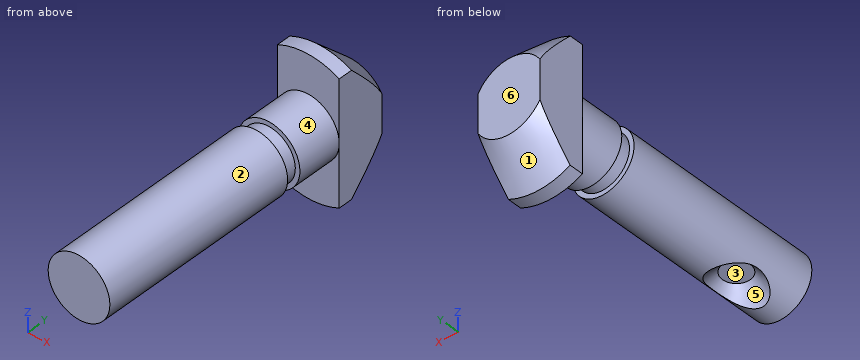
from build123d import *

# Parameters (mm, degrees)
SKETCH_3_W          = 7.345326746
SKETCH_3_H          = 8.819653772
SKETCH_3_W_2        = 8.702196558
SKETCH_3_H_2        = 9.976983905
CUT_EXTRUDE_1_DEPTH = 50


with BuildPart() as part:
    # 草图1 → 旋转1 (revolve)
    with BuildSketch(Plane.XY, mode=Mode.PRIVATE) as revolve_1_sk:
        Polygon((3.95, 33.2), (0, 33.2), (0, 0), (3.35, 0), (3.35, 21.7), (2.85, 21.7), (2.85, 23.2), (3.35, 23.2), (3.35, 28), (7.5, 28), (7.5, 29.5), align=None)
    revolve(revolve_1_sk.sketch.rotate(Axis((0, 33.2, 0), (0, 1, 0)), 270), axis=Axis((0, 33.2, 0), (0, 1, 0)))

    # 草图3 → 切除-拉伸1 (cut, symmetric)
    with BuildSketch(Plane.XY):
        with Locations((-7.022663373, 29.230861624)):
            Rectangle(SKETCH_3_W, SKETCH_3_H)
        with Locations((7.701098279, 29.530171142)):
            Rectangle(SKETCH_3_W_2, SKETCH_3_H_2)
    extrude(amount=CUT_EXTRUDE_1_DEPTH, both=True, mode=Mode.SUBTRACT)

    # 草图4 → 切除-旋转1 (revolve, cut)
    with BuildSketch(Plane(origin=(0, 0, 0), x_dir=(0, 0, -1), z_dir=(1, 0, 0)), mode=Mode.PRIVATE) as cut_revolve_1_sk:
        Polygon((3.35, 5.440830549), (1.65, 5.440830549), (1.65, 6.940830549), (3.35, 8.640830549), align=None)
    revolve(cut_revolve_1_sk.sketch.rotate(Axis((0, 5.440830549, -3.35), (0, 0, 1)), 90), axis=Axis((0, 5.440830549, -3.35), (0, 0, 1)), mode=Mode.SUBTRACT)


solid = part.part
Geometry check sheet. Reference: the model listing, model coordinates, mm. Face numbers are marked on the shaded views. A direction names the side the tool comes from. Round coordinates to 2 decimals unless told otherwise and drop trailing zeros. Loops run counter-clockwise (first coordinate to the right, second up) from the corner with the lowest first, then second, coordinate; pieces in that order, holes last. Notation, with made-up numbers: (52.5, 41) -> (105.5, 41) arc R22 ccw to (105.5, 62) -> close; hole circle Ø2 at (83.5, -33.75). An arc over 180 degrees is marked (long way). Answer as a JSON object with one key per item and string values. Group by question number.
Item 1: Cross-section at A-A, the plane x = 0. Record the cut outline in (y, z), plus the area to 3 significant figures.
Item 2: Thickness scan on line 1 along Y through (x, z) = (2, -2.5); line 2 along X through (y, z) = (16, -0.5); line 3 along Y through (x, z) = (-2, -4.5). Record the ranges inside material, lowest first.
Item 3: Cross-section at D-D, the plane y = 31.5. Record the cut outline in (x, z), plus the area to 3 significant figures.
Item 4: Release check for a two-part mould opening along X. For the marked faces 4, 5 and 6 record: pulls with the +X half, pulls with the -X half, needs draft (parallel to the pull), parting line crosses it, or undercut.
Item 5: Cross-section at C-C, the plane y = 24. Record the cut outline in (x, z), plus the area to 3 significant figures.
Item 6: Depth check by flat-ended pin: pin 1 Ø4 at (x, y) = (-0.5, 14.5) entering from -Z; pin 2 Ø2 at (x, z) = (1, -5) entering from -Y; pin 3 Ø0.9 at (x, y) = (0.5, 5) entering from -Z. Enter the tip coordinate at first touch or a pass-through.
Item 7: Set-up check for the marked faces 1, 2 and 3: record each of +Z, -Z, +X, -X, +Y, -Y from which the full face is reachable in a straight line by a thin tool's end or side.
Determined:
{
 "1": {"outline": "(0, -3.35) -> (2.24, -3.35) -> (3.94, -1.65) -> (6.94, -1.65) -> (8.64, -3.35) -> (21.7, -3.35) -> (21.7, -2.85) -> (23.2, -2.85) -> (23.2, -3.35) -> (28, -3.35) -> (28, -7.5) -> (29.5, -7.5) -> (33.2, -3.95) -> (33.2, 3.95) -> (29.5, 7.5) -> (28, 7.5) -> (28, 3.35) -> (23.2, 3.35) -> (23.2, 2.85) -> (21.7, 2.85) -> (21.7, 3.35) -> (0, 3.35) -> close", "area": "243 mm²"},
 "2": {"line 1": "y = 0 to 4.21, 6.67 to 21.7, 23.2 to 33.2", "line 2": "x = -3.31 to 3.31", "line 3": "y = 28 to 32.18"},
 "3": {"outline": "(-3.35, -4.46) arc R5.58 ccw to (3.35, -4.46) -> (3.35, 4.46) arc R5.58 ccw to (-3.35, 4.46) -> close", "area": "70.0 mm²"},
 "4": {"face 4": "parting line crosses it", "face 5": "undercut", "face 6": "needs draft"},
 "5": {"outline": "circle Ø6.7 at (0, 0)", "area": "35.3 mm²"},
 "6": {"pin 1": "stops at z = -3.35", "pin 2": "stops at y = 28", "pin 3": "stops at z = -1.65"},
 "7": {"face 1": "-Z, +Y", "face 2": "-Y", "face 3": "-Z"}
}
